```python
from build123d import *

# Parameters (mm, degrees)
F0_R     = 6.25
F1_DEPTH = 10


# Not quite as in the source:
# - a feature names something its author has since deleted; it is built from what else it names


with BuildPart() as f1:
    # F0 (on Top) → F1 (new body)
    with BuildSketch(Plane.XY):
        with BuildLine():
            add(Edge.make_bspline(
                [(4.3301272175, 42.4999999798), (7.3612159322, 4.25), (7.3612159322, 4.25), (38.9711430885, -17.5000001821)],
                knots=[0, 0, 0, 0, 69.2820323028, 69.2820323028, 69.2820323028, 69.2820323028], degree=3))
            ThreePointArc((4.3301272175, 42.4999999798), (2.102e-07, 45), (-4.3301268204, 42.5000000202))
            add(Edge.make_bspline(
                [(-38.9711432521, -17.4999998179), (-7.3612159322, 4.25), (-7.3612159322, 4.25), (-4.3301268204, 42.5000000202)],
                knots=[0, 0, 0, 0, 69.2820323028, 69.2820323028, 69.2820323028, 69.2820323028], degree=3))
            ThreePointArc((-38.9711432521, -17.4999998179), (-38.9711432754, -22.4999998179), (-34.6410162682, -24.9999998382))
            add(Edge.make_bspline(
                [(-34.6410162682, -24.9999998382), (0, -8.5), (0, -8.5), (34.6410160346, -25.0000001618)],
                knots=[0, 0, 0, 0, 69.2820323028, 69.2820323028, 69.2820323028, 69.2820323028], degree=3))
            ThreePointArc((34.6410160346, -25.0000001618), (38.9711430652, -22.5000001821), (38.9711430885, -17.5000001821))
        make_face()
        with BuildLine():
            ThreePointArc((6.7724364928, 6.6621395926), (8.2272413629, 4.7499999534), (9.1558004059, 2.5340321482))
            add(Edge.make_bspline(
                [(9.1558004059, 2.5340321482), (12.4794508791, -1.9849209314), (17.9661663578, -5.9523055453), (27.7128128343, -13.0000001849)],
                knots=[28.2758618531, 28.2758618531, 28.2758618531, 28.2758618531, 50.2294734195, 50.2294734195, 50.2294734195, 50.2294734195], degree=3))
            ThreePointArc((27.7128128343, -13.0000001849), (27.7128128143, -16.0000001849), (25.114736593, -17.5000001676))
            add(Edge.make_bspline(
                [(25.114736593, -17.5000001676), (14.1379308325, -12.5830038779), (7.9587172847, -9.8150611129), (2.3833638843, -9.1961718446)],
                knots=[0, 0, 0, 0, 21.953611623, 21.953611623, 21.953611623, 21.953611623], degree=3))
            ThreePointArc((2.3833638843, -9.1961718446), (-5.39e-08, -9.5), (-2.3833639886, -9.1961718175))
            add(Edge.make_bspline(
                [(-2.3833639886, -9.1961718175), (-7.9587173906, -9.8150610209), (-14.1379309923, -12.5830037018), (-25.1147368265, -17.4999998324)],
                knots=[28.2758618531, 28.2758618531, 28.2758618531, 28.2758618531, 50.2294734195, 50.2294734195, 50.2294734195, 50.2294734195], degree=3))
            ThreePointArc((-25.1147368265, -17.4999998324), (-27.7128130279, -15.9999998151), (-27.7128130079, -12.9999998151))
            add(Edge.make_bspline(
                [(-9.1558003771, 2.534032252), (-12.4794509058, -1.9849207937), (-17.9661664304, -5.9523053189), (-27.7128130079, -12.9999998151)],
                knots=[28.2758617965, 28.2758617965, 28.2758617965, 28.2758617965, 50.2294734195, 50.2294734195, 50.2294734195, 50.2294734195], degree=3))
            ThreePointArc((-9.1558003771, 2.534032252), (-8.227241309, 4.7500000466), (-6.7724364173, 6.6621396694))
            add(Edge.make_bspline(
                [(-2.5980760078, 30.5000000173), (-3.8282353656, 18.5353092472), (-4.5207334885, 11.7999819523), (-6.7724364173, 6.6621396694)],
                knots=[0, 0, 0, 0, 21.9536115664, 21.9536115664, 21.9536115664, 21.9536115664], degree=3))
            ThreePointArc((-2.5980760078, 30.5000000173), (2.136e-07, 32), (2.5980764149, 30.4999999827))
            add(Edge.make_bspline(
                [(2.5980764149, 30.4999999827), (3.8282355979, 18.5353091968), (4.5207336211, 11.7999819066), (6.7724364928, 6.6621395926)],
                knots=[0, 0, 0, 0, 21.953611623, 21.953611623, 21.953611623, 21.953611623], degree=3))
        make_face(mode=Mode.SUBTRACT)
        with BuildLine():
            add(Edge.make_bspline(
                [(6.7724364928, 6.6621395926), (7.4208869274, 5.1825322592), (8.1986480984, 3.8354103774), (9.1558004059, 2.5340321482)],
                knots=[21.953611623, 21.953611623, 21.953611623, 21.953611623, 28.2758618531, 28.2758618531, 28.2758618531, 28.2758618531], degree=3))
            ThreePointArc((9.1558004059, 2.5340321482), (8.2272413629, 4.7499999534), (6.7724364928, 6.6621395926))
        make_face()
        with BuildLine():
            ThreePointArc((-2.3833639886, -9.1961718175), (-5.39e-08, -9.5), (2.3833638843, -9.1961718446))
            add(Edge.make_bspline(
                [(2.3833638843, -9.1961718446), (0.7777611287, -9.0179427274), (-0.7777612284, -9.0179427186), (-2.3833639886, -9.1961718175)],
                knots=[21.953611623, 21.953611623, 21.953611623, 21.953611623, 28.2758618531, 28.2758618531, 28.2758618531, 28.2758618531], degree=3))
        make_face()
        with BuildLine():
            add(Edge.make_bspline(
                [(-6.7724364173, 6.6621396694), (-7.42088687, 5.1825323411), (-8.1986480561, 3.8354104682), (-9.1558003771, 2.534032252)],
                knots=[21.9536115664, 21.9536115664, 21.9536115664, 21.9536115664, 28.2758617965, 28.2758617965, 28.2758617965, 28.2758617965], degree=3))
            ThreePointArc((-6.7724364173, 6.6621396694), (-8.227241309, 4.7500000466), (-9.1558003771, 2.534032252))
        make_face()
        with BuildLine():
            ThreePointArc((2.3833638843, -9.1961718446), (7.5130538698, -5.814122595), (9.5, 0))
            ThreePointArc((9.5, 0), (9.413556816, 1.2786508797), (9.1558004059, 2.5340321482))
            add(Edge.make_bspline(
                [(6.7724364928, 6.6621395926), (7.4208869274, 5.1825322592), (8.1986480984, 3.8354103774), (9.1558004059, 2.5340321482)],
                knots=[21.953611623, 21.953611623, 21.953611623, 21.953611623, 28.2758618531, 28.2758618531, 28.2758618531, 28.2758618531], degree=3))
            ThreePointArc((6.7724364928, 6.6621395926), (5.39e-08, 9.5), (-6.7724364173, 6.6621396694))
            add(Edge.make_bspline(
                [(-6.7724364173, 6.6621396694), (-7.42088687, 5.1825323411), (-8.1986480561, 3.8354104682), (-9.1558003771, 2.534032252)],
                knots=[21.9536115664, 21.9536115664, 21.9536115664, 21.9536115664, 28.2758617965, 28.2758617965, 28.2758617965, 28.2758617965], degree=3))
            ThreePointArc((-9.1558003771, 2.534032252), (-8.2272413629, -4.7499999534), (-2.3833639886, -9.1961718175))
            add(Edge.make_bspline(
                [(2.3833638843, -9.1961718446), (0.7777611287, -9.0179427274), (-0.7777612284, -9.0179427186), (-2.3833639886, -9.1961718175)],
                knots=[21.953611623, 21.953611623, 21.953611623, 21.953611623, 28.2758618531, 28.2758618531, 28.2758618531, 28.2758618531], degree=3))
        make_face()
        Circle(F0_R, mode=Mode.SUBTRACT)
    extrude(amount=F1_DEPTH)


solid = f1.part
```
Source: CAD feature listing. Evaluate the final solid. Frame: model axes, mm. A direction names the side the tool comes from. Round coordinates to 2 decimals unless told otherwise and drop trailing zeros. Answer as a JSON object with one key per item and string values. Group by question number.
(1) Reachability of faces 1 (the cylindrical face through (0, 32, 5)), 2 (the cylindrical face through (-39.007, -22.436, 4.93)) from +Z, -Z, +X, -X, +Y, -Y: full face, straight path, thin tool, end or side. Return the list, or none.
(2) Section query A-A on x = 0. State how many separate pieces and enclosed holes the cut face has, then the cut area to 3 significant figures.
(3) Mould query, pull axis X, two halves, no side actions, for faces 3 (the flat face through (6.1, 2.4, 0)), 4 (the cylindrical face through (38.934, -22.563, 4.93)), 5 (the cylindrical face through (-27.69, -16.04, 4.93)). Classes: +X half, -X half, draft (parallel to the pull), parting line (faces both ways), or undercut.
(4) First-contact query: pin 1 (4 mm diameter, centred on y = 31, z = 4, fed in from -X); pin 2 (5 mm diameter, centred on x = 30, z = 7.5, fed in from -Y); pin 3 (4 mm diameter, centred on y = 16, z = 3, fed in from -X); pin 4 (11 mm diameter, centred on x = 0, y = 0, fed in from -Z). Flat tips, straight axial feed; report the tip coordinate or a pass-through.
(5) Ray query, line 1 (Y direction, x = -1, z = 2.75); line 2 (X direction, y = -4.5, z = 4.75); line 3 (X direction, y = -5, z = 6.5). Return the intervals inside material, ascending. Write a range as [from, to].
Computed values:
{
 "1": {"face 1": "+Z, -Z", "face 2": "+Z, -Z, -X"},
 "2": {"separate pieces": "3", "enclosed holes": "0", "area": "226 mm^2"},
 "3": {"face 3": "draft", "face 4": "+X half", "face 5": "undercut"},
 "4": {"pin 1": "x = -5.47", "pin 2": "y = -23.98", "pin 3": "x = -7.84", "pin 4": "through"},
 "5": {"line 1": "[-12.64, -6.17], [6.17, 9.45], [31.83, 44.9]", "line 2": "[-20.86, -16.29], [-8.37, -4.34], [4.34, 8.37], [16.29, 20.86]", "line 3": "[-21.48, -16.92], [-8.08, -3.75], [3.75, 8.08], [16.92, 21.48]"}
}
